```python
from build123d import *

# Parameters (mm, degrees)
CYLINDER004_R     = 25
CYLINDER004_DEPTH = 5
CYLINDER003_R     = 1.5
CYLINDER003_DEPTH = 5
ARRAY_COUNT       = 3
CYLINDER002_R     = 35
CYLINDER002_DEPTH = 5


with BuildPart() as cylinderboring:
    # Cylinder004 → Cylinder004 (new body)
    with BuildSketch(Plane.XY):
        Circle(CYLINDER004_R)
    extrude(amount=CYLINDER004_DEPTH)


with BuildPart() as fusion145:
    # Cylinder003 → Cylinder003 (new body)
    with BuildSketch(Plane(origin=(0, 30, 0), x_dir=(1, 0, 0), z_dir=(0, 0, 1))):
        Circle(CYLINDER003_R)
    extrude(amount=CYLINDER003_DEPTH)

    # Array: Fusion145 ×3 about axis
    array_axis = Axis((0, 0, 0), (0, 0, 1))


with BuildPart() as fusion145_1:
    add(fusion145.part)
    for i in range(1, ARRAY_COUNT):
        add(fusion145.part.rotate(array_axis, i * 360 / ARRAY_COUNT))

    # Fusion145: union CylinderBoring
    add(cylinderboring.part)


with BuildPart() as cut:
    # Cylinder002 → Cylinder002 (new body)
    with BuildSketch(Plane.XY):
        Circle(CYLINDER002_R)
    extrude(amount=CYLINDER002_DEPTH)

    # Cut: cut Fusion145
    add(fusion145_1.part, mode=Mode.SUBTRACT)


solid = cut.part
```
Design review of the part built by this model. Coordinates are the model's own, in mm. Give positions to 0.01 mm unless a question says otherwise; leave off trailing zeros. Order: outer loops, then holes, each group sorted by start corner. A loop starts at its lowest first (then second) coordinate and runs counter-clockwise, first axis right, second up. Notation, with made-up numbers: (-21, 77.5) -> (7, 77.5) arc R19 cw to (7, 99.5) -> close; hole circle Ø6 at (25, 59). An arc over 180 degrees is marked (long way). Write each question's results on one line, items separated by ' | '. Start each with the question number.
Q1. Add section B-B on y = 30. Give the boundary of the cut face in (x, z).
Q2. Mouldability with a two-part tool opening along X and no side actions: class faces 1 (the cylindrical face through (-27.171, -15.913, 2.465)), 2 (the cylindrical face through (24.875, -13.986, 2.465)), 3 (the flat face through (-24, 8, 5)), 4 (the cylindrical face through (-28, -21, 2)) as +X half, -X half, draft (parallel to the pull), parting line (faces both ways), or undercut.
Q3. Add section A-A on x = 0. Give the boundary of the cut face in (y, z), and give its area (3 significant figures).
Q4. Add section D-D on x = 19. Give the boundary of the cut face in (y, z), and give its area (3 significant figures).
Q5. For pin 1 (1.8 mm diameter, centred on x = 0, y = 30, fed in from +Z); pin 2 (1.5 mm diameter, centred on y = -21, z = 3, fed in from -X); pin 3 (1 mm diameter, centred on x = -17, z = 2.5, fed in from +Y), all flat-tipped, find the tip position at first contact; note any pin that passes through.
Q6. Wall thickness on L1, parallel to Y at x = 0, z = 3.9; L2, parallel to Y at x = 22, z = 0.9; L3, parallel to X at y = -8.5, z = 1.1: over which ranges is each line inside the solid? List them lowest first. Write a range as from..to.
Q7. Add section C-C on y = -15. Give the boundary of the cut face in (x, z), and give its area (3 significant figures).
Found:
1) outline: (-18.03, 0) -> (-1.5, 0) -> (-1.5, 5) -> (-18.03, 5) -> close; (1.5, 0) -> (18.03, 0) -> (18.03, 5) -> (1.5, 5) -> close
2) face 1: undercut | face 2: undercut | face 3: draft | face 4: parting line
3) outline: (-35, 0) -> (-25, 0) -> (-25, 5) -> (-35, 5) -> close; (25, 0) -> (28.5, 0) -> (28.5, 5) -> (25, 5) -> close; (31.5, 0) -> (35, 0) -> (35, 5) -> (31.5, 5) -> close | area: 85.0 mm2
4) outline: (-29.39, 0) -> (-16.25, 0) -> (-16.25, 5) -> (-29.39, 5) -> close; (16.25, 0) -> (29.39, 0) -> (29.39, 5) -> (16.25, 5) -> close | area: 131 mm2
5) pin 1: passes through | pin 2: stops at x = -28.55 | pin 3: stops at y = 30.87
6) L1: y = -35..-25, 25..28.5, 31.5..35 | L2: y = -27.22..-11.87, 11.87..27.22 | L3: x = -33.95..-23.51, 23.51..33.95
7) outline: (-31.62, 0) -> (-27.48, 0) -> (-27.48, 5) -> (-31.62, 5) -> close; (-24.48, 0) -> (-20, 0) -> (-20, 5) -> (-24.48, 5) -> close; (20, 0) -> (24.48, 0) -> (24.48, 5) -> (20, 5) -> close; (27.48, 0) -> (31.62, 0) -> (31.62, 5) -> (27.48, 5) -> close | area: 86.2 mm2
